Can you work these out from the model? Positions are in its coordinate system, mm. Face numbers are marked on the shaded views. A direction names the side the tool comes from. Coordinates: 2 decimals unless noted, no trailing zeros. Order: outer loops, then holes, each group sorted by start corner. A loop starts at its lowest first (then second) coordinate and runs counter-clockwise, first axis right, second up. Notation, with made-up numbers: (22, 2) - (52, 2) arc R18 cw to (52, 33) - close; hole circle Ø5 at (4.5, -23). An arc over 180 degrees is marked (long way). Return JSON: item names as keys, results as strings. Group by question number.
1) For pin 1 Ø0.5 at (x, z) = (-1, 9) entering from -Y; pin 2 Ø0.5 at (x, y) = (-1, 0) entering from +Z; pin 3 Ø0.8 at (x, y) = (3.5, 1) entering from +Z, each with a flat end and sliding along its axis, tell me the tip position at first contact or that it passes through.
2) If we mould it in two halves opening along X, with no side actions, what happens to the marked faces 1, 2 and 3? For each: pulls with the +X half, pulls with the -X half, needs draft (parallel to the pull), parting line crosses it, or undercut.
3) Imagine slicing it at D-D (y = 1.25). Write out the boundary of the cut face in (x, z), and give its area (3 significant figures).
4) Which directions (+Z, -Z, +X, -X, +Y, -Y) give clear straight access to the entire face, cutting with the end or side of a thin tool? Please do the marked faces 4, 5 and 6.
5) Imagine slicing it at A-A (z = 3.75). Write out the boundary of the cut face in (x, y), and give its area (3 significant figures).
6) Imagine slicing it at B-B (y = 4.75). Write out the boundary of the cut face in (x, z), and give its area (3 significant figures).
7) If I drill on line 1 along X through (y, z) = (2, 3.5); line 2 along Z through (x, y) = (0.5, 4.5); line 3 along X through (y, z) = (10.25, 4.5), over which ranges is the centre line in solid material (lowest first)?
8) Imagine slicing it at C-C (x = 0.75). Write out the boundary of the cut face in (y, z), and give its area (3 significant figures).
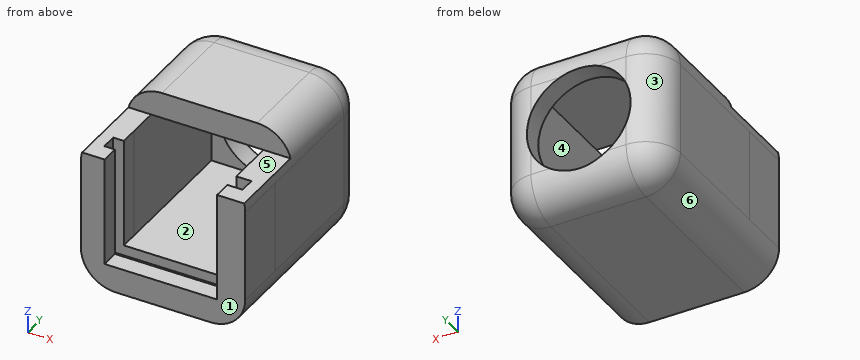
```python
from build123d import *

# Parameters (mm, degrees)
F0_W         = 1.3692331631
F0_H         = 7.834737435
F0_W_2       = 6.5
F0_H_2       = 0.9
F0_W_3       = 0.6192331631
F0_H_3       = 1.05
F0_H_4       = 1.165262565
F0_W_4       = 0.8807668369
F0_W_5       = 1.6307668369
F1_DEPTH     = 0.9
F2_DEPTH     = 1.5
F3_DEPTH     = 7.8
F5_W         = 9.5
F5_H         = 7.2867757659
F6_DEPTH     = 1.5
F7_R         = 3
F8_DEPTH     = 10.501
F9_T1_DEPTH  = 5.3
F9_T3_DEPTH  = 5.5
F9_T5_DEPTH  = 10.2867757659
F9_T7_DEPTH  = 15
F9_S11_W     = 2
F9_S11_H     = 2
F9_T12_DEPTH = 2
F9_S17_W     = 2
F9_S17_H     = 2
F9_T18_DEPTH = 2
F9_S23_W     = 2
F9_S23_H     = 2
F9_T24_DEPTH = 2
F9_S29_W     = 2
F9_S29_H     = 2
F9_T30_DEPTH = 2


# Not quite as in the source:
# - a fillet or chamfer that OpenCascade refuses, or shapes differently, is made with other operations: its cross-section is extruded or revolved along the edge and cut away or added
# - a feature names something its author has since deleted; it is built from what else it names


with BuildPart() as f1:
    # F0 (on Top) → F1 (new body)
    with BuildSketch(Plane.XY):
        Polygon((-4.75, 1.5), (-4.75, -1.5), (-3.3807668369, -1.5), (-3.3807668369, -0.45), (-4, -0.45), (-4, 0.45), (-3.3807668369, 0.45), (-3.3807668369, 1.5), align=None)
        Polygon((-3.3807668369, -0.45), (-3.3807668369, -1.5), (-3.1192331631, -1.5), (3.1192331631, -1.5), (3.1192331631, -0.45), align=None)
        with Locations((-4.0653834185, 5.4173687175)):
            Rectangle(F0_W, F0_H)
        with Locations((-0.1307668369, 0)):
            Rectangle(F0_W_2, F0_H_2)
        with Locations((-3.6903834185, 0)):
            Rectangle(F0_W_3, F0_H_2)
        with Locations((-0.1307668369, 5.4173687175)):
            Rectangle(F0_W_2, F0_H)
        with Locations((-0.1307668369, 0.975)):
            Rectangle(F0_W_2, F0_H_3)
        with Locations((-4.0653834185, 9.9173687175)):
            Rectangle(F0_W, F0_H_4)
        Polygon((3.1192331631, -0.45), (3.1192331631, -1.5), (3.3807668369, -1.5), (4.75, -1.5), (4.75, 1.5), (3.1192331631, 1.5), (3.1192331631, 0.45), (4, 0.45), (4, -0.45), align=None)
        with Locations((3.5596165815, 0)):
            Rectangle(F0_W_4, F0_H_2)
        with Locations((3.9346165815, 5.4173687175)):
            Rectangle(F0_W_5, F0_H)
        with Locations((-0.1307668369, 9.9173687175)):
            Rectangle(F0_W_2, F0_H_4)
        with Locations((3.9346165815, 9.9173687175)):
            Rectangle(F0_W_5, F0_H_4)
    extrude(amount=F1_DEPTH)

    # F0 (on Top) → F2 (join)
    with BuildSketch(Plane.XY):
        Polygon((-3.3807668369, -0.45), (-3.3807668369, -1.5), (-3.1192331631, -1.5), (3.1192331631, -1.5), (3.1192331631, -0.45), align=None)
        Polygon((3.1192331631, -0.45), (3.1192331631, -1.5), (3.3807668369, -1.5), (4.75, -1.5), (4.75, 1.5), (3.1192331631, 1.5), (3.1192331631, 0.45), (4, 0.45), (4, -0.45), align=None)
        Polygon((-4.75, 1.5), (-4.75, -1.5), (-3.3807668369, -1.5), (-3.3807668369, -0.45), (-4, -0.45), (-4, 0.45), (-3.3807668369, 0.45), (-3.3807668369, 1.5), align=None)
        with Locations((-0.1307668369, 0.975)):
            Rectangle(F0_W_2, F0_H_3)
        with Locations((-4.0653834185, 5.4173687175)):
            Rectangle(F0_W, F0_H)
        with Locations((3.9346165815, 5.4173687175)):
            Rectangle(F0_W_5, F0_H)
        with Locations((-0.1307668369, 5.4173687175)):
            Rectangle(F0_W_2, F0_H)
        with Locations((-4.0653834185, 9.9173687175)):
            Rectangle(F0_W, F0_H_4)
        with Locations((-0.1307668369, 9.9173687175)):
            Rectangle(F0_W_2, F0_H_4)
        with Locations((3.9346165815, 9.9173687175)):
            Rectangle(F0_W_5, F0_H_4)
    extrude(amount=F2_DEPTH)

    # F0 (on Top) → F3 (join)
    with BuildSketch(Plane.XY):
        Polygon((-4.75, 1.5), (-4.75, -1.5), (-3.3807668369, -1.5), (-3.3807668369, -0.45), (-4, -0.45), (-4, 0.45), (-3.3807668369, 0.45), (-3.3807668369, 1.5), align=None)
        Polygon((3.1192331631, -0.45), (3.1192331631, -1.5), (3.3807668369, -1.5), (4.75, -1.5), (4.75, 1.5), (3.1192331631, 1.5), (3.1192331631, 0.45), (4, 0.45), (4, -0.45), align=None)
        with Locations((-4.0653834185, 5.4173687175)):
            Rectangle(F0_W, F0_H)
        with Locations((3.9346165815, 5.4173687175)):
            Rectangle(F0_W_5, F0_H)
        with Locations((-4.0653834185, 9.9173687175)):
            Rectangle(F0_W, F0_H_4)
        with Locations((-0.1307668369, 9.9173687175)):
            Rectangle(F0_W_2, F0_H_4)
        with Locations((3.9346165815, 9.9173687175)):
            Rectangle(F0_W_5, F0_H_4)
    extrude(amount=F3_DEPTH)

    # F5 (on offset) → F6 (join)
    with BuildSketch(Plane.XY.offset(7.8)):
        with Locations((0, 6.856612117)):
            Rectangle(F5_W, F5_H)
    extrude(amount=F6_DEPTH)

    # F7 (on Front) → F8 (cut, through all)
    with BuildSketch(Plane.XZ):
        with Locations((0, 4.5)):
            Circle(F7_R)
    extrude(amount=-F8_DEPTH, mode=Mode.SUBTRACT)

    # F9: fillet of radius 2 on 8 edges, made by hand

    # F9_s2 → F9_t1 (cut)
    with BuildSketch(Plane.XY.offset(2)):
        with BuildLine():
            ThreePointArc((4.75, 8.5), (4.1642135624, 9.9142135624), (2.75, 10.5))
            Line((2.75, 10.5), (4.75, 10.5))
            Line((4.75, 10.5), (4.75, 8.5))
        make_face()
        with BuildLine():
            ThreePointArc((-4.75, 8.5), (-4.1642135624, 9.9142135624), (-2.75, 10.5))
            Line((-2.75, 10.5), (-4.75, 10.5))
            Line((-4.75, 10.5), (-4.75, 8.5))
        make_face()
    extrude(amount=F9_T1_DEPTH, mode=Mode.SUBTRACT)

    # F9_s4 → F9_t3 (cut)
    with BuildSketch(Plane.YZ.offset(-2.75)):
        with BuildLine():
            ThreePointArc((8.5, 9.3), (9.9142135624, 8.7142135624), (10.5, 7.3))
            Line((10.5, 7.3), (10.5, 9.3))
            Line((10.5, 9.3), (8.5, 9.3))
        make_face()
        with BuildLine():
            ThreePointArc((8.5, 0), (9.9142135624, 0.5857864376), (10.5, 2))
            Line((10.5, 2), (10.5, 0))
            Line((10.5, 0), (8.5, 0))
        make_face()
    extrude(amount=F9_T3_DEPTH, mode=Mode.SUBTRACT)

    # F9_s6 → F9_t5 (cut)
    with BuildSketch(Plane.XZ.offset(-8.5)):
        with BuildLine():
            ThreePointArc((4.75, 7.3), (4.1642135624, 8.7142135624), (2.75, 9.3))
            Line((2.75, 9.3), (4.75, 9.3))
            Line((4.75, 9.3), (4.75, 7.3))
        make_face()
        with BuildLine():
            ThreePointArc((-4.75, 7.3), (-4.1642135624, 8.7142135624), (-2.75, 9.3))
            Line((-2.75, 9.3), (-4.75, 9.3))
            Line((-4.75, 9.3), (-4.75, 7.3))
        make_face()
    extrude(amount=F9_T5_DEPTH, mode=Mode.SUBTRACT)

    # F9_s8 → F9_t7 (cut)
    with BuildSketch(Plane.XZ.offset(-8.5)):
        with BuildLine():
            ThreePointArc((2.75, 0), (4.1642135624, 0.5857864376), (4.75, 2))
            Line((4.75, 2), (4.75, 0))
            Line((4.75, 0), (2.75, 0))
        make_face()
        with BuildLine():
            ThreePointArc((-4.75, 2), (-4.1642135624, 0.5857864376), (-2.75, 0))
            Line((-2.75, 0), (-4.75, 0))
            Line((-4.75, 0), (-4.75, 2))
        make_face()
    extrude(amount=F9_T7_DEPTH, mode=Mode.SUBTRACT)


with BuildPart() as f9_tool10:
    # F9_s11 → F9_t12 (new body)
    with BuildSketch(Plane.YZ.offset(2.75)):
        with Locations((9.5, 8.3)):
            Rectangle(F9_S11_W, F9_S11_H)
    extrude(amount=F9_T12_DEPTH)

    # F9_s13 → F9_t14 (revolve, cut)
    with BuildSketch(Plane(origin=(2.75, 8.5, 7.3), x_dir=(0, -0.7071067812, -0.7071067812), z_dir=(0, -0.7071067812, 0.7071067812))):
        with BuildLine():
            ThreePointArc((0, -2), (2, 0), (0, 2))
            Line((0, 2), (0, -2))
        make_face()
    revolve(axis=Axis((2.75, 8.5, 7.3), (1, 0, 0)), mode=Mode.SUBTRACT)


with BuildPart() as f1_1:
    add(f1.part)

    # F9_t9: cut F9_tool10
    add(f9_tool10.part, mode=Mode.SUBTRACT)


with BuildPart() as f9_tool16:
    # F9_s17 → F9_t18 (new body)
    with BuildSketch(Plane.XY.offset(2)):
        with Locations((3.75, 9.5)):
            Rectangle(F9_S17_W, F9_S17_H)
    extrude(amount=-F9_T18_DEPTH)

    # F9_s19 → F9_t20 (revolve, cut)
    with BuildSketch(Plane(origin=(2.75, 8.5, 2), x_dir=(-0.7071067812, -0.7071067812, 0), z_dir=(0.7071067812, -0.7071067812, 0))):
        with BuildLine():
            ThreePointArc((0, -2), (2, 0), (0, 2))
            Line((0, 2), (0, -2))
        make_face()
    revolve(axis=Axis((2.75, 8.5, 2), (0, 0, -1)), mode=Mode.SUBTRACT)


with BuildPart() as f1_2:
    add(f1_1.part)

    # F9_t15: cut F9_tool16
    add(f9_tool16.part, mode=Mode.SUBTRACT)


with BuildPart() as f9_tool22:
    # F9_s23 → F9_t24 (new body)
    with BuildSketch(Plane.YZ.offset(-2.75)):
        with Locations((9.5, 8.3)):
            Rectangle(F9_S23_W, F9_S23_H)
    extrude(amount=-F9_T24_DEPTH)

    # F9_s25 → F9_t26 (revolve, cut)
    with BuildSketch(Plane(origin=(-2.75, 8.5, 7.3), x_dir=(0, -0.7071067812, -0.7071067812), z_dir=(0, 0.7071067812, -0.7071067812))):
        with BuildLine():
            ThreePointArc((0, -2), (2, 0), (0, 2))
            Line((0, 2), (0, -2))
        make_face()
    revolve(axis=Axis((-2.75, 8.5, 7.3), (-1, 0, 0)), mode=Mode.SUBTRACT)


with BuildPart() as f1_3:
    add(f1_2.part)

    # F9_t21: cut F9_tool22
    add(f9_tool22.part, mode=Mode.SUBTRACT)


with BuildPart() as f9_tool28:
    # F9_s29 → F9_t30 (new body)
    with BuildSketch(Plane.YZ.offset(-2.75)):
        with Locations((9.5, 1)):
            Rectangle(F9_S29_W, F9_S29_H)
    extrude(amount=-F9_T30_DEPTH)

    # F9_s31 → F9_t32 (revolve, cut)
    with BuildSketch(Plane(origin=(-2.75, 8.5, 2), x_dir=(0, -0.7071067812, 0.7071067812), z_dir=(0, -0.7071067812, -0.7071067812))):
        with BuildLine():
            ThreePointArc((0, -2), (2, 0), (0, 2))
            Line((0, 2), (0, -2))
        make_face()
    revolve(axis=Axis((-2.75, 8.5, 2), (-1, 0, 0)), mode=Mode.SUBTRACT)


with BuildPart() as f1_4:
    add(f1_3.part)

    # F9_t27: cut F9_tool28
    add(f9_tool28.part, mode=Mode.SUBTRACT)


solid = f1_4.part
```
Calculated:
{
 "1": {"pin 1": "y = 3.21", "pin 2": "z = 0.9", "pin 3": "z = 7.8"},
 "2": {"face 1": "needs draft", "face 2": "undercut", "face 3": "pulls with the -X half"},
 "3": {"outline": "(-4.75, 2) arc R2 ccw to (-2.75, 0) - (2.75, 0) arc R2 ccw to (4.75, 2) - (4.75, 7.3) arc R2 ccw to (4.69, 7.8) - (3.12, 7.8) - (3.12, 1.5) - (-3.38, 1.5) - (-3.38, 7.8) - (-4.69, 7.8) arc R2 ccw to (-4.75, 7.3) - close", "area": "31.4 mm2"},
 "4": {"face 4": "-Y", "face 5": "+Z, +X, -X, -Y", "face 6": "-Z, -X, +Y, -Y"},
 "5": {"outline": "(-4.75, -1.5) - (-3.38, -1.5) - (-3.38, -0.45) - (-4, -0.45) - (-4, 0.45) - (-3.38, 0.45) - (-3.38, 9.33) - (-2.9, 9.33) - (-2.9, 10.49) arc R2 ccw to (-4.75, 8.5) - close; (2.9, 9.33) - (3.12, 9.33) - (3.12, 0.45) - (4, 0.45) - (4, -0.45) - (3.12, -0.45) - (3.12, -1.5) - (4.75, -1.5) - (4.75, 8.5) arc R2 ccw to (2.9, 10.49) - close", "area": "33.7 mm2"},
 "6": {"outline": "(-4.75, 2) arc R2 ccw to (-2.75, 0) - (2.75, 0) arc R2 ccw to (4.75, 2) - (4.75, 7.3) arc R2 ccw to (2.75, 9.3) - (-2.75, 9.3) arc R2 ccw to (-4.75, 7.3) - close; hole (-3.38, 1.5) - (3.12, 1.5) - (3.12, 7.8) - (-3.38, 7.8) - close", "area": "44.0 mm2"},
 "7": {"line 1": "-4.75 to -3.38, 3.12 to 4.75", "line 2": "0 to 1.5, 7.8 to 9.3", "line 3": "-3.72 to -3, 3 to 3.72"},
 "8": {"outline": "(-1.5, 0) - (8.5, 0) arc R2 ccw to (10.46, 1.6) - (9.33, 1.6) - (9.33, 1.5) - (0.45, 1.5) - (0.45, 0.9) - (-0.45, 0.9) - (-0.45, 1.5) - (-1.5, 1.5) - close; (3.21, 7.8) - (9.33, 7.8) - (9.33, 7.4) - (10.5, 7.4) arc R2 ccw to (8.5, 9.3) - (3.21, 9.3) - close", "area": "27.3 mm2"}
}
